```python
from build123d import *

# Parameters (mm, degrees)
SKETCH_1_W               = 14
SKETCH_1_H               = 13.200286042
EXTRUDE_1_DEPTH          = 3
SKETCH_3_OUTSIDE_W       = 35.048
SKETCH_3_OUTSIDE_H       = 82.027
CUT_EXTRUDE_2_DEPTH      = 3
SKETCH_4_R               = 3
CUT_EXTRUDE_3_DEPTH      = 10
SKETCH_5_R               = 1
CUT_EXTRUDE_4_DEPTH      = 10
SKETCH_6_W               = 4
SKETCH_6_H               = 4
EXTRUDE_3_DEPTH          = 3
CUT_EXTRUDE_5_DEPTH      = 10
PATTERN_CIRCULAR_1_COUNT = 8
SKETCH_9_W               = 14
SKETCH_9_H               = 26
EXTRUDE_4_DEPTH          = 11
CUT_EXTRUDE_8_DEPTH      = 7
SKETCH_11_R              = 10
CUT_EXTRUDE_9_DEPTH      = 7
SKETCH_12_W              = 4
SKETCH_12_H              = 4
CUT_EXTRUDE_10_DEPTH     = 1


with BuildPart() as part:
    # 草图1 → 凸台-拉伸1 (new body)
    with BuildSketch(Plane.XY):
        Rectangle(SKETCH_1_W, SKETCH_1_H)
        with BuildLine():
            ThreePointArc((-7, 6.600143021), (-9.620908892, 0), (-7, -6.600143021))
            Line((-7, -6.600143021), (-7, 6.600143021))
        make_face()
        with BuildLine():
            Line((7, -6.600143021), (-7, -6.600143021))
            ThreePointArc((-7, -6.600143021), (0, -9.620908892), (7, -6.600143021))
        make_face()
        with BuildLine():
            Line((7, 6.600143021), (7, -6.600143021))
            ThreePointArc((7, -6.600143021), (8.941707056, -3.550741166), (9.620908892, 0))
            ThreePointArc((9.620908892, 0), (8.941707056, 3.550741166), (7, 6.600143021))
        make_face()
        with BuildLine():
            ThreePointArc((7, 6.600143021), (0, 9.620908892), (-7, 6.600143021))
            Line((-7, 6.600143021), (7, 6.600143021))
        make_face()
        with BuildLine():
            Line((-7, 56.600143021), (-7, 6.600143021))
            ThreePointArc((-7, 6.600143021), (0, 9.620908892), (7, 6.600143021))
            Line((7, 6.600143021), (7, 56.600143021))
            Line((7, 56.600143021), (-7, 56.600143021))
        make_face()
    extrude(amount=EXTRUDE_1_DEPTH)

    # 草图3 outside → 切除-拉伸2 (cut)
    with BuildSketch(Plane.XY.offset(3)):
        with Locations((0, 23.4895)):
            Rectangle(SKETCH_3_OUTSIDE_W, SKETCH_3_OUTSIDE_H)
        with BuildLine():
            Line((7, 56.600143021), (0, 56.600143021))
            Line((0, 56.600143021), (-7, 56.600143021))
            Line((-7, 56.600143021), (-7, 6.600143021))
            ThreePointArc((-7, 6.600143021), (0, -9.620908892), (7, 6.600143021))
            Line((7, 6.600143021), (7, 56.600143021))
        make_face(mode=Mode.SUBTRACT)
        Polygon((-2, 28.600143021), (0, 28.600143021), (2, 28.600143021), (2, 24.600143021), (-2, 24.600143021), align=None)
        Polygon((-2, 38.600143021), (0, 38.600143021), (2, 38.600143021), (2, 34.600143021), (0, 34.600143021), (-2, 34.600143021), align=None)
        Polygon((-2, 48.600143021), (0, 48.600143021), (2, 48.600143021), (2, 44.600143021), (0, 44.600143021), (-2, 44.600143021), align=None)
    extrude(amount=-CUT_EXTRUDE_2_DEPTH, mode=Mode.SUBTRACT)

    # 草图4 → 切除-拉伸3 (cut)
    with BuildSketch(Plane.XY.offset(3)):
        Circle(SKETCH_4_R)
    extrude(amount=-CUT_EXTRUDE_3_DEPTH, mode=Mode.SUBTRACT)

    # 草图5 → 切除-拉伸4 (cut)
    with BuildSketch(Plane(origin=(0, 0, 0), x_dir=(-1, 0, 0), z_dir=(0, 0, -1))):
        with Locations((0, 6.5)):
            Circle(SKETCH_5_R)
    cut_extrude_4 = extrude(amount=-CUT_EXTRUDE_4_DEPTH, mode=Mode.SUBTRACT)

    # 草图6 → 凸台-拉伸3 (add)
    with BuildSketch(Plane(origin=(0, 0, 0), x_dir=(-1, 0, 0), z_dir=(0, 0, -1))):
        with Locations((0, 36.600143021)):
            Rectangle(SKETCH_6_W, SKETCH_6_H)
    extrude(amount=-EXTRUDE_3_DEPTH)

    # 草图7 → 切除-拉伸5 (cut)
    with BuildSketch(Plane(origin=(0, 0, 0), x_dir=(-1, 0, 0), z_dir=(0, 0, -1))):
        with BuildLine():
            ThreePointArc((0, 38.600143021), (-2, 36.600143021), (0, 34.600143021))
            Line((0, 34.600143021), (0, 38.600143021))
        make_face()
        with BuildLine():
            Line((0, 38.600143021), (0, 34.600143021))
            ThreePointArc((0, 34.600143021), (1.414213562, 35.185929459), (2, 36.600143021))
            ThreePointArc((2, 36.600143021), (1.414213562, 38.014356584), (0, 38.600143021))
        make_face()
    extrude(amount=-CUT_EXTRUDE_5_DEPTH, mode=Mode.SUBTRACT)

    # 阵列(圆周)1: 切除-拉伸4 ×8 about axis
    pattern_circular_1_axis = Axis((0, 0, 0), (0, 0, 1))
    for i in range(1, PATTERN_CIRCULAR_1_COUNT):
        add(cut_extrude_4.rotate(pattern_circular_1_axis, i * 360 / PATTERN_CIRCULAR_1_COUNT), mode=Mode.SUBTRACT)

    # 草图9 → 凸台-拉伸4 (add)
    with BuildSketch(Plane.XY.offset(3)):
        with Locations((0, 36.600143021)):
            Rectangle(SKETCH_9_W, SKETCH_9_H)
    extrude(amount=EXTRUDE_4_DEPTH)

    # 草图10 → 切除-拉伸8 (cut)
    with BuildSketch(Plane.ZY.offset(7)):
        Polygon((4, 36.618598328), (9.5, 27.092318886), (14, 27.092318886), (14, 46.14487777), (9.5, 46.14487777), align=None)
    extrude(amount=-CUT_EXTRUDE_8_DEPTH, mode=Mode.SUBTRACT)

    # 草图11 → 切除-拉伸9 (cut)
    with BuildSketch(Plane.ZY):
        with Locations((14, 36.618598328)):
            Circle(SKETCH_11_R)
    extrude(amount=-CUT_EXTRUDE_9_DEPTH, mode=Mode.SUBTRACT)

    # 草图12 → 切除-拉伸10 (cut)
    with BuildSketch(Plane(origin=(0, 0, 3), x_dir=(-1, 0, 0), z_dir=(0, 0, -1))):
        with Locations((0, 46.600143021)):
            Rectangle(SKETCH_12_W, SKETCH_12_H)
        with Locations((0, 26.600143021)):
            Rectangle(SKETCH_12_W, SKETCH_12_H)
    extrude(amount=-CUT_EXTRUDE_10_DEPTH, mode=Mode.SUBTRACT)


solid = part.part
```
Read the model definition and answer for the solid it produces. Units are mm, in the model's axes. A direction names the side the tool comes from. Give positions to 0.01 mm unless a question says otherwise; leave off trailing zeros. Order: outer loops, then holes, each group sorted by start corner. A loop starts at its lowest first (then second) coordinate and runs counter-clockwise, first axis right, second up. Notation, with made-up numbers: (-13.75, -30) -> (33.25, -30) arc R27 cw to (33.25, -5) -> close; hole circle Ø1 at (11, 88.5). An arc over 180 degrees is marked (long way). One line per item, written item: value. Start each with the question number.
(1) The part is cut by section A-A (z = 12.5). Determine the outline of the cut face in (x, y), and give its area (3 significant figures).
(2) A tool of negligible diameter and unlimited length cuts with its end or side. For faces 3 (the flat face through (-4, 46.145, 12)), 4 (the flat face through (2, 27, 2)), 5 (the flat face through (0, 41, 6)), 6 (the cylindrical face through (3.75, -4.06, 1.48)), from which of +Z, -Z, +X, -X, +Y, -Y can it reach the whole face along a straight path? Write none if from no direction.
(3) Straight lines are drawn through the part: L1, parallel to Y at x = 4, z = 0.75; L2, parallel to X at y = 26.5, z = 2.25; L3, parallel to X at y = 45.5, z = 6. For each, find the intervals that lie inside material, in ascending order.
(4) The part is cut by section C-C (y = 10). Determine the outline of the cut face in (x, z), and give its area (3 significant figures).
(5) The part is cut by section D-D (z = 8.25). Determine the outline of the cut face in (x, y), and give its area (3 significant figures).
(6) Flat-ended cylindrical pins translate along their axes: P1, Ø2, axis at y = 27, z = 2.5, coming from the +X side; P2, Ø6, axis at y = 46, z = 11, coming from the -X side; P3, Ø1.5, axis at x = 4.5, z = 9.5, coming from the +Y side. Find the tip coordinate at first contact, or state that the pin passes through.
(7) The part is cut by section B-B (z = 1). State how many separate pieces and enclosed holes the cut face has, and give its area (3 significant figures).
(8) For a pull along X with two mould halves and no side action, classify faces 1 (the flat face through (-2, 27, 2)), 2 (the flat face through (0, 53, 3)) as released by +X, released by -X, zero draft, split by the parting line, or undercut.
Taken from the geometry:
1. outline: (-7, 23.6) -> (7, 23.6) -> (7, 26.73) -> (0, 26.73) -> (0, 27.09) -> (-7, 27.09) -> close; (-7, 46.14) -> (0, 46.14) -> (0, 46.51) -> (7, 46.51) -> (7, 49.6) -> (-7, 49.6) -> close
1. area: 92.2 mm^2
2. face 3: +Z, -X
2. face 4: -Z
2. face 5: +Z, +X
2. face 6: +Z, -Z
3. L1: -8.75 to -5.4, -3.79 to 3.79, 5.4 to 56.6
3. L2: -7 to -2, 2 to 7
3. L3: -7 to 7
4. outline: (-7, 0) -> (7, 0) -> (7, 3) -> (-7, 3) -> close
4. area: 42.0 mm^2
5. outline: (-7, 23.6) -> (7, 23.6) -> (7, 28.44) -> (0, 28.44) -> (0, 29.26) -> (-7, 29.26) -> close; (-7, 43.98) -> (0, 43.98) -> (0, 44.8) -> (7, 44.8) -> (7, 49.6) -> (-7, 49.6) -> close
5. area: 146 mm^2
6. P1: x = 7
6. P2: x = -7
6. P3: y = 49.6
7. separate pieces: 1
7. enclosed holes: 12
7. area: 864 mm^2
8. face 1: undercut
8. face 2: zero draft
